from build123d import *

# Parameters (mm, degrees)
F0_W     = 60.619533062
F0_H     = 48.4413802624
F1_DEPTH = 560
F2_DEPTH = 600
F3_DEPTH = 720
F4_T     = -18


with BuildPart() as f1:
    # F0 (on Front) → F1 (new body)
    with BuildSketch(Plane.XZ):
        with Locations((30.309766531, 24.2206901312)):
            Rectangle(F0_W, F0_H)
    extrude(amount=-F1_DEPTH)

    # F2 (add): a face of the model
    f2_faces = [f1.faces().sort_by_distance(p)[0] for p in [
        (0, 280, 24.2206901312),
    ]]
    extrude(f2_faces, amount=-F2_DEPTH)

    # F3 (add): a face of the model
    f3_faces = [f1.faces().sort_by_distance(p)[0] for p in [
        (300, 280, 0),
    ]]
    extrude(f3_faces, amount=-F3_DEPTH)

    # F4
    f4_openings = [f1.faces().sort_by_distance(p)[0] for p in [
        (300, 560, 360),
        (300, 280, 720),
    ]]
    offset(amount=F4_T, openings=f4_openings)


solid = f1.part
The listing builds one solid part. Answer for the finished solid, in the listing's coordinates (mm). A direction names the side the tool comes from. Round coordinates to 2 decimals unless told otherwise and drop trailing zeros. Write each loop counter-clockwise with the first axis right and the second up, starting at its lowest first coordinate (ties: lowest second). Pieces come first, ordered by that corner, then holes. Notation, with made-up numbers: M 78,12 L 84,12 A24 cw 84,31 Z; hole C 49.5,63 d1. An arc over 180 degrees is marked long. Write each question's results on one line, items separated by ' | '. Start each with the question number.
(1) For faces 1 (the flat face through (296, 276, 0)), 2 (the flat face through (296, 18, 374)), determine the directions among +Z, -Z, +X, -X, +Y, -Y from which every point of the face is accessible in a straight line to the end or side of a thin tool.
(2) The part is cut by section A-A, the plane z = 386.5. Write down the section's boundary in (x, y), and give its area (3 significant figures).
(3) Determine the mould class of faces 3 (the flat face through (0, 276, 355)), 4 (the flat face through (18, 285, 364)), 5 (the flat face through (582, 285, 364)), 6 (the flat face through (296, 0, 365)) for opening direction X: +X half, -X half, draft (parallel to the pull), parting line (faces both ways), or undercut.
(4) Find the intervals of material crossed by line 1 (X direction, y = 163, z = 571.5); line 2 (Y direction, x = 374, z = 403.5), in increasing order.
(5) The part is cut by section C-C, the plane x = 150.5. Write down the section's boundary in (y, z).
(6) Each of these flat-tipped pins is pushed along its axis until it touches: P1, Ø2, axis at x = 278.5, y = 497.5, coming from the +Z side; P2, Ø2, axis at x = 459, z = 593.5, coming from the +Y side. Where does it stop, or does it pass through?
(7) The part is cut by section B-B, the plane y = 320. Write down the section's boundary in (x, z), and give its area (3 significant figures).
Worked answers:
1) face 1: -Z, +X, -X, +Y, -Y | face 2: +Z, +Y
2) outline: M 0,0 L 600,0 L 600,560 L 582,560 L 582,18 L 18,18 L 18,560 L 0,560 Z | area: 30,300 mm²
3) face 3: -X half | face 4: undercut | face 5: undercut | face 6: draft
4) line 1: x = 0 to 18, 582 to 600 | line 2: y = 0 to 18
5) outline: M 0,0 L 560,0 L 560,18 L 18,18 L 18,720 L 0,720 Z
6) P1: stops at z = 18 | P2: stops at y = 18
7) outline: M 0,0 L 600,0 L 600,720 L 582,720 L 582,18 L 18,18 L 18,720 L 0,720 Z | area: 36,100 mm²
